The listing builds one solid part. Answer for the finished solid, in the listing's coordinates (mm). A direction names the side the tool comes from. Coordinates: 2 decimals unless noted, no trailing zeros. Write each loop counter-clockwise with the first axis right and the second up, starting at its lowest first coordinate (ties: lowest second). Pieces come first, ordered by that corner, then holes.
from build123d import *

# Parameters (mm, degrees)
SKETCH1_W           = 2
SKETCH1_H           = 40
MAIN_ANGLE          = 90
SUPPORT_DEPTH       = 12
SKETCH6_W           = 1
SKETCH6_H           = 2.9
FIX_2_DEPTH         = 12
SKETCH9_R           = 1.6
SKETCH9_W           = 60
SKETCH9_H           = 8
HOLES_DEPTH         = 7
SKETCH10_R          = 4.25
BIGHOLES_DEPTH      = 30.5
REINFORCEMENT_DEPTH = 10
SKETCH12_W          = 70.003571338
SKETCH12_H          = 12
SENSORWINDOW_DEPTH  = 35.5000001


with BuildPart() as part:
    # Sketch1 → Main (revolve, symmetric)
    with BuildSketch(Plane.XY) as main_sk:
        with Locations((48.5, 20)):
            Rectangle(SKETCH1_W, SKETCH1_H)
    revolve(axis=Axis((0, -0.284703924, 0), (0, 1, 0)), revolution_arc=MAIN_ANGLE / 2)
    revolve(main_sk.sketch, axis=Axis((0, -0.284703924, 0), (0, -1, 0)), revolution_arc=MAIN_ANGLE / 2)

    # Sketch2 → Support (add)
    with BuildSketch(Plane(origin=(0, 10, 0), x_dir=(-1, 0, 0), z_dir=(0, -1, 0))):
        with BuildLine():
            Line((-43.957365708, -18), (-20, -18))
            Line((-20, -18), (-20, 18))
            Line((-20, 18), (-43.957365708, 18))
            ThreePointArc((-43.957365708, 18), (-40.835530357, 24.263335724), (-36.827299657, 30))
            Line((-36.827299657, 30), (-15, 30))
            Line((-15, 30), (-15, -30))
            Line((-15, -30), (-36.827299657, -30))
            ThreePointArc((-36.827299657, -30), (-40.835530357, -24.263335724), (-43.957365708, -18))
        make_face()
    extrude(amount=-SUPPORT_DEPTH)

    # Sketch6 → Fix 2 (add)
    with BuildSketch(Plane(origin=(0, 10, 0), x_dir=(1, 0, 0), z_dir=(0, 1, 0))):
        with Locations((14.5, -25)):
            Rectangle(SKETCH6_W, SKETCH6_H)
        with Locations((14.5, 25)):
            Rectangle(SKETCH6_W, SKETCH6_H)
    extrude(amount=FIX_2_DEPTH)

    # Sketch9 → Holes (cut, through all)
    with BuildSketch(Plane(origin=(20, 0, 0), x_dir=(0, 0, -1), z_dir=(1, 0, 0))):
        with Locations((25, 16)):
            Circle(SKETCH9_R)
        with Locations((-25, 16)):
            Circle(SKETCH9_R)
        with Locations((0, 38)):
            Rectangle(SKETCH9_W, SKETCH9_H)
    extrude(amount=-HOLES_DEPTH, mode=Mode.SUBTRACT)

    # Sketch10 → BigHoles (cut, through all)
    with BuildSketch(Plane(origin=(20, 0, 0), x_dir=(0, 0, -1), z_dir=(1, 0, 0))):
        with Locations((25, 16)):
            Circle(SKETCH10_R)
        with Locations((-25, 16)):
            Circle(SKETCH10_R)
    extrude(amount=BIGHOLES_DEPTH, mode=Mode.SUBTRACT)

    # Sketch11 → Reinforcement (add)
    with BuildSketch(Plane(origin=(0, 22, 0), x_dir=(1, 0, 0), z_dir=(0, 1, 0))):
        Polygon((20, 18), (25, 18), (20, 13), align=None)
        Polygon((20, -18), (20, -13), (25, -18), align=None)
        Polygon((41.111278447, 18), (46.111278447, 18), (46.111278447, 13), align=None)
        Polygon((41.111278447, -18), (46.111278447, -18), (46.111278447, -11.401754251), align=None)
    extrude(amount=-REINFORCEMENT_DEPTH)

    # Sketch12 → SensorWindow (cut, through all)
    with BuildSketch(Plane.ZY.offset(-15)):
        with Locations((0, 34)):
            Rectangle(SKETCH12_W, SKETCH12_H)
    extrude(amount=-SENSORWINDOW_DEPTH, mode=Mode.SUBTRACT)


solid = part.part
1. Section C-C on x = 17.5 is taken. Give the vertices of the cut face in (y, z).
Results found:
outline: (10, -30) - (22, -30) - (22, 30) - (10, 30) - close; hole circle Ø3.2 at (16, -25); hole circle Ø3.2 at (16, 25)
2. For a pull along Z with two mould halves and no side action, classify faces 1 (the flat face through (48, 28, 0)), 2 (the flat face through (15, 16, 0)) as pulls with the +Z half, pulls with the -Z half, needs draft (parallel to the pull), parting line crosses it, or undercut.
Results found:
face 1: needs draft
face 2: undercut
3. Section B-B on y = 16 is taken. State how many separate pieces and enclosed holes the cut face has, then the cut area to 3 significant figures.
Results found:
separate pieces: 3
enclosed holes: 1
area: 576 mm2
4. Find the intervals of material crossed by L1, parallel to Z at x = 31, y = 16; L2, parallel to Y at x = 18, z = 25; L3, parallel to Y at x = 28, z = 25, in increasing order.
Results found:
L1: z = -30 to -29.25, -20.75 to -18, 18 to 20.75, 29.25 to 30
L2: y = 10 to 14.4, 17.6 to 22
L3: y = 10 to 11.75, 20.25 to 22
5. Section D-D on z = 25 is taken. Give the vertices of the cut face in (x, y), then the cut area to 3 significant figures.
Results found:
outline: (14, 10) - (40.39, 10) - (40.39, 0) - (42.72, 0) - (42.72, 11.75) - (20, 11.75) - (20, 14.4) - (14, 14.4) - close; (14, 17.6) - (20, 17.6) - (20, 20.25) - (42.72, 20.25) - (42.72, 28) - (40.39, 28) - (40.39, 22) - (14, 22) - close
area: 170 mm2
6. Section A-A on x = 31.5 is taken. Give the vertices of the cut face in (y, z), then the cut area to 3 significant figures.
Results found:
outline: (10, -30) - (22, -30) - (22, -18) - (10, -18) - close; (10, 18) - (22, 18) - (22, 30) - (10, 30) - close; hole circle Ø8.5 at (16, -25); hole circle Ø8.5 at (16, 25)
area: 175 mm2
7. Flat-ended cylindrical pins translate along their axes: P1, Ø3, axis at y = 13.5, z = 4.5, coming from the +X side; P2, Ø8, axis at y = 7, z = -13.5, coming from the -X side; P3, Ø3, axis at x = 18, z = 9, coming from the -Y side. Find the tip coordinate at first contact, or state that the pin passes through.
Results found:
P1: stops at x = 49.41
P2: stops at x = 15
P3: stops at y = 10
8. A tool of negligible diameter and unlimited length cuts with its end or side. For faces 3 (the flat face through (20, 16, -27)), 4 (the flat face through (19, 10, 0)), 5 (the flat face through (15, 16, 28)), from which of +Z, -Z, +X, -X, +Y, -Y can it reach the whole face along a straight path? Write none if from no direction.
Results found:
face 3: +X
face 4: -X, -Y
face 5: +Z, -X, +Y, -Y
